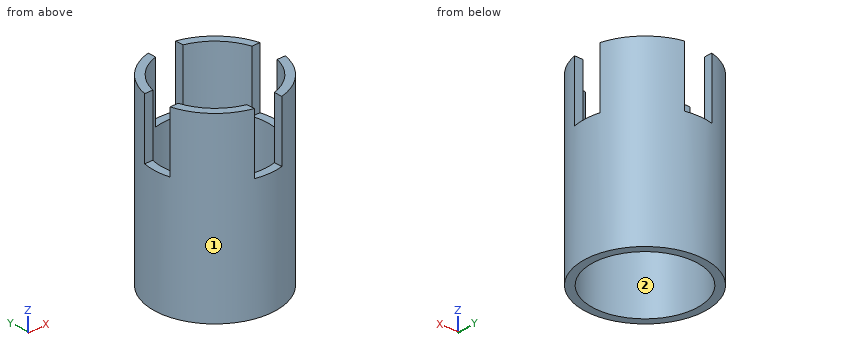
from build123d import *

# Parameters (mm, degrees)
F0_R     = 15.1
F0_R_2   = 13.1
F1_DEPTH = 45
F2_W     = 7
F2_H     = 15
F3_DEPTH = 25
F4_DEPTH = 25
F5_W     = 7
F5_H     = 15
F6_DEPTH = 25
F7_DEPTH = 25


with BuildPart() as f1:
    # F0 (on Top) → F1 (new body)
    with BuildSketch(Plane.XY):
        Circle(F0_R)
        Circle(F0_R_2, mode=Mode.SUBTRACT)
    extrude(amount=F1_DEPTH)

    # F2 (on Front) → F3 (cut)
    with BuildSketch(Plane.XZ):
        with Locations((0, 37.5)):
            Rectangle(F2_W, F2_H)
    extrude(amount=-F3_DEPTH, mode=Mode.SUBTRACT)

    # F2 (on Front) → F4 (cut)
    with BuildSketch(Plane.XZ):
        with Locations((0, 37.5)):
            Rectangle(F2_W, F2_H)
    extrude(amount=F4_DEPTH, mode=Mode.SUBTRACT)

    # F5 (on Right) → F6 (cut)
    with BuildSketch(Plane.YZ):
        with Locations((0, 37.5)):
            Rectangle(F5_W, F5_H)
    extrude(amount=-F6_DEPTH, mode=Mode.SUBTRACT)

    # F5 (on Right) → F7 (cut)
    with BuildSketch(Plane.YZ):
        with Locations((0, 37.5)):
            Rectangle(F5_W, F5_H)
    extrude(amount=F7_DEPTH, mode=Mode.SUBTRACT)


solid = f1.part
Build history of the part. All positions in model axes, mm. Face numbers are marked on the shaded views. Coordinates: 2 decimals unless noted, no trailing zeros. Write each loop counter-clockwise with the first axis right and the second up, starting at its lowest first coordinate (ties: lowest second). Pieces come first, ordered by that corner, then holes.
(1) Cut at A-A on y = 0. List the corners of the cut face in (x, z).
(2) Mould opens along X. For the marked faces 1 and 2 say: pulls with the +X half, pulls with the -X half, needs draft (parallel to the pull), parting line crosses it, or undercut.
(3) Pin check, flat tips, straight feed: pin 1 Ø6 at (x, z) = (-7, 27.5) entering from -Y; pin 2 Ø1 at (x, z) = (-5.5, 28.5) entering from +Y; pin 3 Ø1 at (x, z) = (-13.5, 38) entering from +Y; pin 4 Ø10 at (x, y) = (-6.5, 1.5) entering from +Z. Stop position of each tip, or through.
(4) Cut at C-C on z = 9.5. List the corners of the cut face in (x, y), and give its area (3 significant figures).
(5) Drill centre lines: line 1 (Y direction, x = 0, z = 10); line 2 (X direction, y = -12, z = 10.5); line 3 (Y direction, x = 2, z = 14.5). Where is each one in solid material? Low to high.
Working result:
1. outline: (-15.1, 0) - (-13.1, 0) - (-13.1, 30) - (-15.1, 30) - close; (13.1, 0) - (15.1, 0) - (15.1, 30) - (13.1, 30) - close
2. face 1: parting line crosses it
2. face 2: undercut
3. pin 1: stops at y = -14.56
3. pin 2: stops at y = 14.25
3. pin 3: stops at y = 7.68
3. pin 4: passes through
4. outline: circle Ø30.2 at (0, 0); hole circle Ø26.2 at (0, 0)
4. area: 177 mm2
5. line 1: y = -15.1 to -13.1, 13.1 to 15.1
5. line 2: x = -9.17 to -5.25, 5.25 to 9.17
5. line 3: y = -14.97 to -12.95, 12.95 to 14.97
